Read the model definition and answer for the solid it produces. Units are mm, in the model's axes. A direction names the side the tool comes from. Coordinates: 2 decimals unless noted, no trailing zeros. Loops run counter-clockwise (first coordinate to the right, second up) from the corner with the lowest first, then second, coordinate; pieces in that order, holes last. Notation, with made-up numbers: (48, 74) -> (67, 74) arc R8 ccw to (67, 78) -> close; hole circle Ø6 at (-1, 15). An arc over 180 degrees is marked (long way). One line per question, with ' | ' between items. Start each with the question number.
```python
from build123d import *

# Parameters (mm, degrees)
F0_W     = 61
F0_H     = 34.1
F1_DEPTH = 2
F3_DEPTH = 3
F4_D     = 3.4


with BuildPart() as f1:
    # F0 (on Top) → F1 (new body)
    with BuildSketch(Plane.XY):
        Rectangle(F0_W, F0_H)
    extrude(amount=F1_DEPTH)

    # F2 (on face) → F3 (join)
    with BuildSketch(Plane.XY.offset(2)):
        with BuildLine():
            Line((-24.7, 17.05), (-30.5, 17.05))
            Line((-30.5, 17.05), (-30.5, 11.25))
            Line((-30.5, 11.25), (-25.7, 11.25))
            ThreePointArc((-25.7, 11.25), (-24.9928932188, 11.5428932188), (-24.7, 12.25))
            Line((-24.7, 12.25), (-24.7, 17.05))
        make_face()
        with BuildLine():
            Line((-25.7, -11.25), (-30.5, -11.25))
            Line((-30.5, -11.25), (-30.5, -17.05))
            Line((-30.5, -17.05), (-24.7, -17.05))
            Line((-24.7, -17.05), (-24.7, -12.25))
            ThreePointArc((-24.7, -12.25), (-24.9928932188, -11.5428932188), (-25.7, -11.25))
        make_face()
        with BuildLine():
            Line((30.5, -17.05), (30.5, -11.25))
            Line((30.5, -11.25), (25.7, -11.25))
            ThreePointArc((25.7, -11.25), (24.9928932188, -11.5428932188), (24.7, -12.25))
            Line((24.7, -12.25), (24.7, -17.05))
            Line((24.7, -17.05), (30.5, -17.05))
        make_face()
        with BuildLine():
            Line((30.5, 17.05), (24.7, 17.05))
            Line((24.7, 17.05), (24.7, 12.25))
            ThreePointArc((24.7, 12.25), (24.9928932188, 11.5428932188), (25.7, 11.25))
            Line((25.7, 11.25), (30.5, 11.25))
            Line((30.5, 11.25), (30.5, 17.05))
        make_face()
    extrude(amount=F3_DEPTH)

    # F4 (through all)
    with Locations(Plane(origin=(0, 0, 0), x_dir=(1, 0, 0), z_dir=(0, 0, -1))):
        with Locations((-27.6, -14.15), (27.6, -14.15), (27.6, 14.15), (-27.6, 14.15)):
            Hole(F4_D / 2)


solid = f1.part
```
(1) Section A-A on x = -27.6 is taken. Write down the section's boundary in (y, z), plus the area to 3 significant figures.
(2) A tool of negligible diameter and unlimited length cuts with its end or side. For faces 4 (the flat face through (0, -17.05, 1)), 5 (the flat face through (24.7, 15, 3)), 6 (the flat face through (-28, 11.25, 3)), 7 (the flat face through (0, 0, 2)), from which of +Z, -Z, +X, -X, +Y, -Y can it reach the whole face along a straight path? Write none if from no direction.
(3) Find the intervals of material crossed by probe 1 along X at (y, z) = (14.15, 3); probe 2 along Y at (x, z) = (27.6, 1.1); probe 3 along X at (y, z) = (14.15, 1.8), in increasing order. Write a range as from..to.
(4) Section D-D on y = -1.5 is taken. Write down the section's boundary in (x, z), plus the area to 3 significant figures.
(5) Section C-C on x = -5.5 is taken. Write down the section's boundary in (y, z).
(6) Section B-B on y = 14.15 is taken. Write down the section's boundary in (x, z), plus the area to 3 significant figures.
(7) Determine the mould class of faces 1 (the flat face through (30.5, 0, 1)), 2 (the flat face through (-26, -13, 5)), 3 (the flat face through (-24.7, 15, 3)) for opening direction X: +X half, -X half, draft (parallel to the pull), parting line (faces both ways), or undercut.
(8) Each of these flat-tipped pins is pushed along its axis until it touches: pin 1 Ø12 at (x, y) = (-6, -0.5) entering from +Z; pin 2 Ø1 at (y, z) = (10.5, 4) entering from +X. Where does it stop, or does it pass through?
Working result:
1) outline: (-17.05, 0) -> (-15.85, 0) -> (-15.85, 5) -> (-17.05, 5) -> close; (-12.45, 0) -> (12.45, 0) -> (12.45, 5) -> (11.25, 5) -> (11.25, 2) -> (-11.25, 2) -> (-11.25, 5) -> (-12.45, 5) -> close; (15.85, 0) -> (17.05, 0) -> (17.05, 5) -> (15.85, 5) -> close | area: 69.0 mm2
2) face 4: +Z, -Z, +X, -X, -Y | face 5: +Z, +Y, -Y | face 6: +Z, +X, -X | face 7: +Z
3) probe 1: x = -30.5..-29.3, -25.9..-24.7, 24.7..25.9, 29.3..30.5 | probe 2: y = -17.05..-15.85, -12.45..12.45, 15.85..17.05 | probe 3: x = -30.5..-29.3, -25.9..25.9, 29.3..30.5
4) outline: (-30.5, 0) -> (30.5, 0) -> (30.5, 2) -> (-30.5, 2) -> close | area: 122 mm2
5) outline: (-17.05, 0) -> (17.05, 0) -> (17.05, 2) -> (-17.05, 2) -> close
6) outline: (-30.5, 0) -> (-29.3, 0) -> (-29.3, 5) -> (-30.5, 5) -> close; (-25.9, 0) -> (25.9, 0) -> (25.9, 5) -> (24.7, 5) -> (24.7, 2) -> (-24.7, 2) -> (-24.7, 5) -> (-25.9, 5) -> close; (29.3, 0) -> (30.5, 0) -> (30.5, 5) -> (29.3, 5) -> close | area: 123 mm2
7) face 1: +X half | face 2: draft | face 3: undercut
8) pin 1: stops at z = 2 | pin 2: passes through
